from build123d import *

# Parameters (mm, degrees)
SKETCH_1_R            = 1.6
SKETCH_1_R_2          = 1.1
F_85_1P5MM_DEPTH      = 1.5
CUT_EXTRUDE_384_DEPTH = 1.5


with BuildPart() as part:
    # 草图1 → 85方雷达盖板_1p5mm (new body)
    with BuildSketch(Plane.XY):
        Polygon((-42.5, -39.5), (-39.5, -42.5), (39.5, -42.5), (42.5, -39.5), (42.5, 39.5), (39.5, 42.5), (-39.5, 42.5), (-42.5, 39.5), align=None)
        with Locations((-24, -18)):
            Circle(SKETCH_1_R, mode=Mode.SUBTRACT)
        with Locations((-24, 18)):
            Circle(SKETCH_1_R, mode=Mode.SUBTRACT)
        with Locations((24, -18)):
            Circle(SKETCH_1_R, mode=Mode.SUBTRACT)
        with Locations((24, 18)):
            Circle(SKETCH_1_R, mode=Mode.SUBTRACT)
        with Locations((-21, -39)):
            Circle(SKETCH_1_R_2, mode=Mode.SUBTRACT)
        with Locations((-8, -39)):
            Circle(SKETCH_1_R_2, mode=Mode.SUBTRACT)
        with Locations((8, -39)):
            Circle(SKETCH_1_R_2, mode=Mode.SUBTRACT)
        with Locations((21, -39)):
            Circle(SKETCH_1_R_2, mode=Mode.SUBTRACT)
    extrude(amount=F_85_1P5MM_DEPTH)

    # 草图4 → Cut-Extrude 384 (cut)
    with BuildSketch(Plane.XY):
        Polygon((-12, -12), (12, -12), (16, -8), (16, 8), (12, 12), (-12, 12), (-16, 8), (-16, -8), align=None)
        Polygon((-32, -21), (-36, -21), (-38, -19), (-38, 19), (-36, 21), (-32, 21), (-30, 19), (-30, -19), align=None)
        Polygon((32, -21), (36, -21), (38, -19), (38, 19), (36, 21), (32, 21), (30, 19), (30, -19), align=None)
        Polygon((-12, -22), (12, -22), (14, -24), (14, -28), (12, -30), (-12, -30), (-14, -28), (-14, -24), align=None)
        Polygon((-12, 22), (12, 22), (14, 24), (14, 28), (12, 30), (-12, 30), (-14, 28), (-14, 24), align=None)
    extrude(amount=CUT_EXTRUDE_384_DEPTH, mode=Mode.SUBTRACT)


solid = part.part
Input: part model. Units: mm. Frame: model coordinates. Give positions to 0.01 mm unless a question says otherwise; leave off trailing zeros. Write each loop counter-clockwise with the first axis right and the second up, starting at its lowest first coordinate (ties: lowest second). Pieces come first, ordered by that corner, then holes. Notation, with made-up numbers: M -35.75,74.25 L 5.25,74.25 A28 cw 5.25,113.25 Z; hole C 61.5,53 d4. An arc over 180 degrees is marked long. Write item = value, one per line. Start each with the question number.
1) Cut plane A-A on y = -7. Return the cut outline in (x, z).
2) Cut plane D-D on y = 18. Return the cut outline in (x, z), then the cut area to 3 significant figures.
3) Cut plane C-C on x = 37. Return the cut outline in (y, z), then the cut area to 3 significant figures.
4) Draft query along X for faces 1 (the flat face through (41, -41, 1)), 2 (the cylindrical face through (23.792, -16.414, 0.74)). Return one class per face: +X half, -X half, draft (parallel to the pull), parting line (faces both ways), or undercut.
5) Cut plane B-B on x = -13. Return the cut outline in (y, z).
6) First-contact query: pin 1 Ø1 at (x, y) = (14.5, -34) entering from -Z; pin 2 Ø1.9 at (x, y) = (24, 18) entering from -Z. Flat tips, straight axial feed; report the tip coordinate or a pass-through.
7) Material intervals for line 1 along Y through (x, z) = (24, 0.95); line 2 along X through (y, z) = (-5, 1.2); line 3 along X through (y, z) = (25, 0.15), sorted ascending. Write a range as [from, to].
Solved:
q1.outline = M -42.5,0 L -38,0 L -38,1.5 L -42.5,1.5 Z; M -30,0 L -16,0 L -16,1.5 L -30,1.5 Z; M 16,0 L 30,0 L 30,1.5 L 16,1.5 Z; M 38,0 L 42.5,0 L 42.5,1.5 L 38,1.5 Z
q2.outline = M -42.5,0 L -38,0 L -38,1.5 L -42.5,1.5 Z; M -30,0 L -25.6,0 L -25.6,1.5 L -30,1.5 Z; M -22.4,0 L 22.4,0 L 22.4,1.5 L -22.4,1.5 Z; M 25.6,0 L 30,0 L 30,1.5 L 25.6,1.5 Z; M 38,0 L 42.5,0 L 42.5,1.5 L 38,1.5 Z
q2.area = 93.9 mm2
q3.outline = M -42.5,0 L -20,0 L -20,1.5 L -42.5,1.5 Z; M 20,0 L 42.5,0 L 42.5,1.5 L 20,1.5 Z
q3.area = 67.5 mm2
q4.face_1 = +X half
q4.face_2 = undercut
q5.outline = M -42.5,0 L -29,0 L -29,1.5 L -42.5,1.5 Z; M -23,0 L -11,0 L -11,1.5 L -23,1.5 Z; M 11,0 L 23,0 L 23,1.5 L 11,1.5 Z; M 29,0 L 42.5,0 L 42.5,1.5 L 29,1.5 Z
q6.pin_1 = 0
q6.pin_2 = through
q7.line_1 = [-42.5, -19.6], [-16.4, 16.4], [19.6, 42.5]
q7.line_2 = [-42.5, -38], [-30, -16], [16, 30], [38, 42.5]
q7.line_3 = [-42.5, -14], [14, 42.5]
